Autodesk Inventor part; units mm, degrees
sketch "Sketch1" plane through (0, 0, 0) normal (0, 0, 1) x (1, 0, 0)
  line L0 (50, -50) -> (-50, -50)
  line L1 (-50, -50) -> (-50, 50)
  line L2 (-50, 50) -> (50, 50)
  line L3 (50, 50) -> (50, -50)
  line L4 (50, -50) -> (-50, 50) construction
  line L5 (-50, -50) -> (50, 50) construction
  line L6 (-40, 40) -> (-40, -40)
  line L7 (-40, -40) -> (40, -40)
  line L8 (40, -40) -> (40, 40)
  line L9 (40, 40) -> (-40, 40)
  point P0 (0, 0)
  dimension "d0" = 100
  dimension "d1" = 100
  dimension "d2" = 10
extrude "Extrusion1" add sketch "Sketch1" along normal mid plane 750
properties part number "Perna_001_0001" material "Steel"
Geometry: final body of the model. Coordinates: model frame, mm. A direction names the side the tool comes from. Give positions to 0.01 mm unless a question says otherwise; leave off trailing zeros. Write each loop counter-clockwise with the first axis right and the second up, starting at its lowest first coordinate (ties: lowest second). Pieces come first, ordered by that corner, then holes.
(1) Access query for faces 1 (the flat face through (40, -1, -5)), 2 (the flat face through (-1, 50, -5)). Directions: +Z, -Z, +X, -X, +Y, -Y. A direction counts if a zero-diameter tool reaches every point of the face in a straight line with its end or side. Return the directions, or none.
(2) Ray query, line 1 (Y direction, x = 10, z = -8.5). Return the intervals inside material, ascending.
(3) Cut plane C-C, the plane z = 206.5. Return loops of the section in (x, y), then the cut area to 3 significant figures.
(4) Mould query, pull axis Y, two halves, no side actions, for faces 3 (the flat face through (-1, -40, -5)), 4 (the flat face through (-45, 1, 375)), 5 (the flat face through (1, -50, -5)). Classes: released by +Y, released by -Y, zero draft, split by the parting line, or undercut.
(5) Cut plane A-A, the plane y = -3.5. Return loops of the section in (x, z).
Values follow:
1. face 1: +Z, -Z
1. face 2: +Z, -Z, +X, -X, +Y
2. line 1: y = -50 to -40, 40 to 50
3. outline: (-50, -50) - (50, -50) - (50, 50) - (-50, 50) - close; hole (-40, -40) - (40, -40) - (40, 40) - (-40, 40) - close
3. area: 3,600 mm2
4. face 3: undercut
4. face 4: zero draft
4. face 5: released by -Y
5. outline: (-50, -375) - (-40, -375) - (-40, 375) - (-50, 375) - close; (40, -375) - (50, -375) - (50, 375) - (40, 375) - close
